Design review of the part built by this model. Coordinates are the model's own, in mm. A direction names the side the tool comes from. Give positions to 0.01 mm unless a question says otherwise; leave off trailing zeros. Loops run counter-clockwise (first coordinate to the right, second up) from the corner with the lowest first, then second, coordinate; pieces in that order, holes last. Notation, with made-up numbers: M -5.5,-31 L 16.5,-31 A19 ccw 16.5,-19 Z; hole C 48.5,62.25 d11. An arc over 180 degrees is marked long. Use a Markdown table: item, result. Add a question column.
(1) Draft analysis for pull direction Z (two halves, no side actions). For faces 5 (the face through (0.49, -15.62, 3.47)), 6 (the face through (0.7, 2.96, -5.22)), 7 (the face through (0.9, -11.9, -1.1)), 8 (the face through (0, -7, -7)), state which applies: pulls with the +Z half, pulls with the -Z half, needs draft (parallel to the pull), parting line crosses it, or undercut.
(2) Add section A-A, the plane x = 0.65. Give the boundary of the cut face in (y, z).
(3) For faces 1 (the face through (0.9, -1.1, 11.5)), 2 (the face through (0.696, 3.042, 5.172)), 3 (the face through (1, -7, 0)), 4 (the face through (0.4, -6.3, 0)), list the 3-axis set-ups (+Z, -Z, +X, -X, +Y, -Y) from which the entire face can be reached by the end or side of a thin tool; tool diameter is ignored.
(4) For probe 1 along Y at (x, z) = (0.55, 1); probe 2 along Y at (x, z) = (0.35, 0); probe 3 along X at (y, z) = (5.5, 6), list the stretches that pass through material, from the lowest coordinate up.
```python
from build123d import *

# Parameters (mm, degrees)
SKETCH1_R           = 16
SKETCH1_R_2         = 8.5
BOSS_EXTRUDE1_DEPTH = 1
SKETCH1_3_R         = 8.5
CUT_EXTRUDE1_DEPTH  = 0.4
CUT_EXTRUDE2_DEPTH  = 0.1


with BuildPart() as part:
    # Sketch1 → Boss-Extrude1 (new body)
    with BuildSketch(Plane(origin=(0, 0, 0), x_dir=(0, 0, -1), z_dir=(1, 0, 0))):
        Circle(SKETCH1_R)
        Circle(SKETCH1_R_2, mode=Mode.SUBTRACT)
        Circle(SKETCH1_R_2)
        Polygon((3.464101615, -6), (6.92820323, 0), (3.464101615, 6), (-3.464101615, 6), (-6.92820323, 0), (-3.464101615, -6), align=None, mode=Mode.SUBTRACT)
    extrude(amount=BOSS_EXTRUDE1_DEPTH)

    # Sketch1_3 → Cut-Extrude1 (cut)
    with BuildSketch(Plane(origin=(0, 0, 0), x_dir=(0, 0, -1), z_dir=(1, 0, 0))):
        Circle(SKETCH1_3_R)
        Polygon((3.464101615, -6), (6.92820323, 0), (3.464101615, 6), (-3.464101615, 6), (-6.92820323, 0), (-3.464101615, -6), align=None, mode=Mode.SUBTRACT)
    extrude(amount=CUT_EXTRUDE1_DEPTH, mode=Mode.SUBTRACT)

    # Sketch2 → Cut-Extrude2 (cut)
    with BuildSketch(Plane(origin=(1, 0, 0), x_dir=(0, 0, -1), z_dir=(1, 0, 0))):
        with BuildLine():
            ThreePointArc((0, 7.778308753), (-0.339285063, 7.770905526), (-0.677924277, 7.74870994))
            add(Edge.make_bspline(
                [(-0.88309199, 16.154115956), (-2.272109381, 12.182110552), (-0.677924277, 7.74870994)],
                knots=[0, 0, 0, 1, 1, 1], degree=2))
            ThreePointArc((-0.88309199, 16.154115956), (-0.611192857, 16.166686645), (-0.33912072, 16.174681169))
            add(Edge.make_bspline(
                [(0, 7.778308753), (-1.708704101, 11.993417261), (-0.33912072, 16.174681169)],
                knots=[0, 0, 0, 1, 1, 1], degree=2))
        make_face()
        with BuildLine():
            ThreePointArc((3.889154376, 6.736212978), (3.59162328, 6.899444127), (3.287255324, 7.049541793))
            add(Edge.make_bspline(
                [(7.312277881, 14.431420789), (4.123350831, 11.6860719), (3.287255324, 7.049541793)],
                knots=[0, 0, 0, 1, 1, 1], degree=2))
            ThreePointArc((7.312277881, 14.431420789), (7.554034782, 14.306357758), (7.793653427, 14.177245151))
            add(Edge.make_bspline(
                [(3.889154376, 6.736212978), (4.516927471, 11.240956077), (7.793653427, 14.177245151)],
                knots=[0, 0, 0, 1, 1, 1], degree=2))
        make_face()
        with BuildLine():
            ThreePointArc((6.736212978, 3.889154376), (6.560159065, 4.179282246), (6.371617516, 4.461454615))
            add(Edge.make_bspline(
                [(13.548328799, 8.841838075), (9.413962519, 8.05875972), (6.371617516, 4.461454615)],
                knots=[0, 0, 0, 1, 1, 1], degree=2))
            ThreePointArc((13.548328799, 8.841838075), (13.695164901, 8.612651864), (13.838124431, 8.381027743))
            add(Edge.make_bspline(
                [(6.736212978, 3.889154376), (9.532251976, 7.47648979), (13.838124431, 8.381027743)],
                knots=[0, 0, 0, 1, 1, 1], degree=2))
        make_face()
        with BuildLine():
            ThreePointArc((7.778308753, 0), (7.770905526, 0.339285063), (7.74870994, 0.677924277))
            add(Edge.make_bspline(
                [(16.154115956, 0.88309199), (12.182110552, 2.272109381), (7.74870994, 0.677924277)],
                knots=[0, 0, 0, 1, 1, 1], degree=2))
            ThreePointArc((16.154115956, 0.88309199), (16.166686645, 0.611192857), (16.174681169, 0.33912072))
            add(Edge.make_bspline(
                [(7.778308753, 0), (11.993417261, 1.708704101), (16.174681169, 0.33912072)],
                knots=[0, 0, 0, 1, 1, 1], degree=2))
        make_face()
        with BuildLine():
            ThreePointArc((6.736212978, -3.889154376), (6.899444127, -3.59162328), (7.049541793, -3.287255324))
            add(Edge.make_bspline(
                [(14.431420789, -7.312277881), (11.6860719, -4.123350831), (7.049541793, -3.287255324)],
                knots=[0, 0, 0, 1, 1, 1], degree=2))
            ThreePointArc((14.431420789, -7.312277881), (14.306357758, -7.554034782), (14.177245151, -7.793653427))
            add(Edge.make_bspline(
                [(6.736212978, -3.889154376), (11.240956077, -4.516927471), (14.177245151, -7.793653427)],
                knots=[0, 0, 0, 1, 1, 1], degree=2))
        make_face()
        with BuildLine():
            ThreePointArc((3.889154376, -6.736212978), (4.179282246, -6.560159065), (4.461454615, -6.371617516))
            add(Edge.make_bspline(
                [(8.841838075, -13.548328799), (8.05875972, -9.413962519), (4.461454615, -6.371617516)],
                knots=[0, 0, 0, 1, 1, 1], degree=2))
            ThreePointArc((8.841838075, -13.548328799), (8.612651864, -13.695164901), (8.381027743, -13.838124431))
            add(Edge.make_bspline(
                [(3.889154376, -6.736212978), (7.47648979, -9.532251976), (8.381027743, -13.838124431)],
                knots=[0, 0, 0, 1, 1, 1], degree=2))
        make_face()
        with BuildLine():
            ThreePointArc((0, -7.778308753), (0.339285063, -7.770905526), (0.677924277, -7.74870994))
            add(Edge.make_bspline(
                [(0.88309199, -16.154115956), (2.272109381, -12.182110552), (0.677924277, -7.74870994)],
                knots=[0, 0, 0, 1, 1, 1], degree=2))
            ThreePointArc((0.88309199, -16.154115956), (0.611192857, -16.166686645), (0.33912072, -16.174681169))
            add(Edge.make_bspline(
                [(0, -7.778308753), (1.708704101, -11.993417261), (0.33912072, -16.174681169)],
                knots=[0, 0, 0, 1, 1, 1], degree=2))
        make_face()
        with BuildLine():
            ThreePointArc((-3.889154376, -6.736212978), (-3.59162328, -6.899444127), (-3.287255324, -7.049541793))
            add(Edge.make_bspline(
                [(-7.312277881, -14.431420789), (-4.123350831, -11.6860719), (-3.287255324, -7.049541793)],
                knots=[0, 0, 0, 1, 1, 1], degree=2))
            ThreePointArc((-7.312277881, -14.431420789), (-7.554034782, -14.306357758), (-7.793653427, -14.177245151))
            add(Edge.make_bspline(
                [(-3.889154376, -6.736212978), (-4.516927471, -11.240956077), (-7.793653427, -14.177245151)],
                knots=[0, 0, 0, 1, 1, 1], degree=2))
        make_face()
        with BuildLine():
            ThreePointArc((-6.736212978, -3.889154376), (-6.560159065, -4.179282246), (-6.371617516, -4.461454615))
            add(Edge.make_bspline(
                [(-13.548328799, -8.841838075), (-9.413962519, -8.05875972), (-6.371617516, -4.461454615)],
                knots=[0, 0, 0, 1, 1, 1], degree=2))
            ThreePointArc((-13.548328799, -8.841838075), (-13.695164901, -8.612651864), (-13.838124431, -8.381027743))
            add(Edge.make_bspline(
                [(-6.736212978, -3.889154376), (-9.532251976, -7.47648979), (-13.838124431, -8.381027743)],
                knots=[0, 0, 0, 1, 1, 1], degree=2))
        make_face()
        with BuildLine():
            ThreePointArc((-7.778308753, 0), (-7.770905526, -0.339285063), (-7.74870994, -0.677924277))
            add(Edge.make_bspline(
                [(-16.154115956, -0.88309199), (-12.182110552, -2.272109381), (-7.74870994, -0.677924277)],
                knots=[0, 0, 0, 1, 1, 1], degree=2))
            ThreePointArc((-16.154115956, -0.88309199), (-16.166686645, -0.611192857), (-16.174681169, -0.33912072))
            add(Edge.make_bspline(
                [(-7.778308753, 0), (-11.993417261, -1.708704101), (-16.174681169, -0.33912072)],
                knots=[0, 0, 0, 1, 1, 1], degree=2))
        make_face()
        with BuildLine():
            ThreePointArc((-6.736212978, 3.889154376), (-6.899444127, 3.59162328), (-7.049541793, 3.287255324))
            add(Edge.make_bspline(
                [(-14.431420789, 7.312277881), (-11.6860719, 4.123350831), (-7.049541793, 3.287255324)],
                knots=[0, 0, 0, 1, 1, 1], degree=2))
            ThreePointArc((-14.431420789, 7.312277881), (-14.306357758, 7.554034782), (-14.177245151, 7.793653427))
            add(Edge.make_bspline(
                [(-6.736212978, 3.889154376), (-11.240956077, 4.516927471), (-14.177245151, 7.793653427)],
                knots=[0, 0, 0, 1, 1, 1], degree=2))
        make_face()
        with BuildLine():
            ThreePointArc((-3.889154376, 6.736212978), (-4.179282246, 6.560159065), (-4.461454615, 6.371617516))
            add(Edge.make_bspline(
                [(-8.841838075, 13.548328799), (-8.05875972, 9.413962519), (-4.461454615, 6.371617516)],
                knots=[0, 0, 0, 1, 1, 1], degree=2))
            ThreePointArc((-8.841838075, 13.548328799), (-8.612651864, 13.695164901), (-8.381027743, 13.838124431))
            add(Edge.make_bspline(
                [(-3.889154376, 6.736212978), (-7.47648979, 9.532251976), (-8.381027743, 13.838124431)],
                knots=[0, 0, 0, 1, 1, 1], degree=2))
        make_face()
    extrude(amount=-CUT_EXTRUDE2_DEPTH, mode=Mode.SUBTRACT)


solid = part.part
```
Established:
| question | item | result |
|---|---|---|
| 1 | face 5 | parting line crosses it |
| 1 | face 6 | undercut |
| 1 | face 7 | undercut |
| 1 | face 8 | needs draft |
| 2 | outline | C 0,0 d32; hole M -6,-3.46 L 0,-6.93 L 6,-3.46 L 6,3.46 L 0,6.93 L -6,3.46 Z |
| 3 | face 1 | +X |
| 3 | face 2 | +X, -X |
| 3 | face 3 | +Z, -Z, +X, +Y, -Y |
| 3 | face 4 | -X |
| 4 | probe 1 | -15.97 to -6, 6 to 15.97 |
| 4 | probe 2 | -16 to -8.5, 8.5 to 16 |
| 4 | probe 3 | 0.4 to 1 |
